Design review of the part built by this model. Coordinates are the model's own, in mm. Give positions to 0.01 mm unless a question says otherwise; leave off trailing zeros. Loops run counter-clockwise (first coordinate to the right, second up) from the corner with the lowest first, then second, coordinate; pieces in that order, holes last.
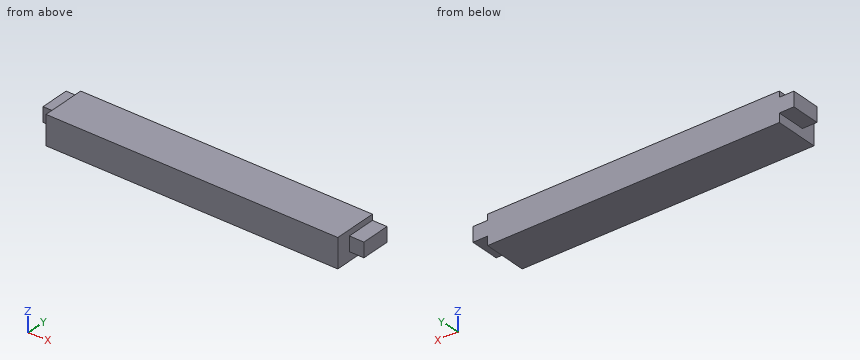
from build123d import *

# Parameters (mm, degrees)
F0_W     = 200
F0_H     = 30
F1_DEPTH = 20
F2_W     = 20
F2_H     = 10
F3_DEPTH = 10


with BuildPart() as f1:
    # F0 (on Top) → F1 (new body)
    with BuildSketch(Plane.XY):
        Rectangle(F0_W, F0_H)
    extrude(amount=F1_DEPTH)

    # F2 (on face) → F3 (join)
    with BuildSketch(Plane.YZ.offset(100)):
        with Locations((5, 11.047103)):
            Rectangle(F2_W, F2_H)
    extrude(amount=F3_DEPTH)

    # F4: F1 across plane


with BuildPart() as f1_1:
    add(f1.part)
    add(f1.part.mirror(Plane.YZ))


with BuildPart() as f5_1:
    # F5: copy of F1
    add(f1_1.part.moved(Location((0, 50, 0))))


solid = f5_1.part
Q1. Take a section at A-A (z = 12.5). Give the boundary of the cut face in (x, y), plus the area to 3 significant figures.
Results:
outline: (-110, 45) - (-100, 45) - (-100, 35) - (100, 35) - (100, 45) - (110, 45) - (110, 65) - (-110, 65) - close
area: 6,400 mm2
Q2. Insertion check: pin 1 (3 mm diameter, centred on y = 44, z = 11, fed in from -X); pin 2 (5 mm diameter, centred on x = -105, y = 52.5, fed in from -Z); pin 3 (3 mm diameter, centred on y = 40, z = 18, fed in from +X); pin 4 (5 mm diameter, centred on x = -107, z = 10, fed in from -Y). Each pin has a flat end and moves straight along its axis. Give the tip position at first contact, or say it passes through.
Results:
pin 1: stops at x = -110
pin 2: stops at z = 6.05
pin 3: stops at x = 100
pin 4: stops at y = 45
Q3. Take a section at C-C (z = 4.25). Give the boundary of the cut face in (x, y), plus the area to 3 significant figures.
Results:
outline: (-100, 35) - (100, 35) - (100, 65) - (-100, 65) - close
area: 6,000 mm2
Q4. Take a section at B-B (y = 56.25). Give the boundary of the cut face in (x, z), plus the area to 3 significant figures.
Results:
outline: (-110, 6.05) - (-100, 6.05) - (-100, 0) - (100, 0) - (100, 6.05) - (110, 6.05) - (110, 16.05) - (100, 16.05) - (100, 20) - (-100, 20) - (-100, 16.05) - (-110, 16.05) - close
area: 4,200 mm2
Q5. Take a section at D-D (y = 37). Give the boundary of the cut face in (x, z), plus the area to 3 significant figures.
Results:
outline: (-100, 0) - (100, 0) - (100, 20) - (-100, 20) - close
area: 4,000 mm2
Q6. Wall thickness on line 1 (X direction, y = 60.75, z = 17): over which ranges is the line inside the solid? List them lowest first.
Results:
line 1: x = -100 to 100
